from build123d import *

# Parameters (mm, degrees)
SKETCH003_W     = 161.5
SKETCH003_H     = 211.5
SKETCH003_W_2   = 130
SKETCH003_H_2   = 180
PAD002_DEPTH    = 18.5
SKETCH004_W     = 142.953762
SKETCH004_H     = 192.038153
SKETCH004_W_2   = 116
SKETCH004_H_2   = 167
PAD003_DEPTH    = 7.6
SKETCH011_W     = 36.28281
SKETCH011_H     = 83.99005
POCKET002_DEPTH = 6.5


with BuildPart() as part:
    # Sketch003 (on XY_Plane031 of Origin062) → Pad002 (new body)
    with BuildSketch(Plane.XY):
        with Locations((80.75, 105.75)):
            Rectangle(SKETCH003_W, SKETCH003_H)
        with Locations((80.75, 105.75)):
            Rectangle(SKETCH003_W_2, SKETCH003_H_2, mode=Mode.SUBTRACT)
    extrude(amount=PAD002_DEPTH)

    # Sketch004 (on Face10 of Pad002) → Pad003 (join)
    with BuildSketch(Plane.XY.offset(18.5)):
        with Locations((79.935823, 103.608654)):
            Rectangle(SKETCH004_W, SKETCH004_H)
        with Locations((80.75, 105.75)):
            Rectangle(SKETCH004_W_2, SKETCH004_H_2, mode=Mode.SUBTRACT)
    extrude(amount=-PAD003_DEPTH)

    # Sketch011 (on Face4 of Pad003) → Pocket002 (cut)
    with BuildSketch(Plane(origin=(0, 0, 0), x_dir=(1, 0, 0), z_dir=(0, 0, -1))):
        with Locations((161.891405, -94.345025)):
            Rectangle(SKETCH011_W, SKETCH011_H)
    extrude(amount=-POCKET002_DEPTH, mode=Mode.SUBTRACT)


solid = part.part
Check sheet for the modelled part. Datum: model origin and axes. Units: mm. A direction names the side the tool comes from. Give positions to 0.01 mm unless a question says otherwise; leave off trailing zeros. Write each loop counter-clockwise with the first axis right and the second up, starting at its lowest first coordinate (ties: lowest second). Pieces come first, ordered by that corner, then holes. Notation, with made-up numbers: (-37, -29) -> (-19, -29) arc R3 cw to (-19, -25) -> close; hole circle Ø11 at (57.5, 42.25). An arc over 180 degrees is marked (long way). One line per item, written item: value. Start each with the question number.
Item 1: Section check B-B on x = 110. Record the cut outline in (y, z), then the cut area to 3 significant figures.
Item 2: Section check C-C on y = 19. Record the cut outline in (x, z), then the cut area to 3 significant figures.
Item 3: Gauge pin test, flat ends, axial feed: pin 1 (5.5 mm diameter, centred on x = 53, z = 4.5, fed in from -Y); pin 2 (17.5 mm diameter, centred on x = 154, y = 113, fed in from -Z). Record the tip position at first contact, or that the pin passes through.
Item 4: Tool access check on faces 1 (the flat face through (0, 104, 9)), 2 (the flat face through (80, 22.25, 15)), 3 (the flat face through (80, 15.75, 5)), 4 (the flat face through (154, 52.35, 3)), 5 (the flat face through (8, 107, 18.5)). Record the directions out of +Z, -Z, +X, -X, +Y, -Y that give a thin tool (end or side, any length) a straight path to the whole face; none if there is none.
Item 5: Section check A-A on y = 42.5. Record the cut outline in (x, z).
Item 6: Section check D-D on x = 151.5. Record the cut outline in (y, z).
Item 7: Draft check along X on faces 6 (the flat face through (161.5, 104, 11)), 7 (the flat face through (80, 189.25, 15)), 8 (the flat face through (154, 94, 6.5)). Enter one of: +X half, -X half, draft (parallel to the pull), parting line (faces both ways), or undercut.
Item 8: Material ranges on probe 1 along Y at (x, z) = (88, 16); probe 2 along Y at (x, z) = (119.5, 1); probe 3 along X at (y, z) = (60, 17.25), recorded low to high. Write a range as from..to.
Results list:
1. outline: (0, 0) -> (15.75, 0) -> (15.75, 10.9) -> (22.25, 10.9) -> (22.25, 18.5) -> (0, 18.5) -> close; (189.25, 10.9) -> (195.75, 10.9) -> (195.75, 0) -> (211.5, 0) -> (211.5, 18.5) -> (189.25, 18.5) -> close
1. area: 682 mm²
2. outline: (0, 0) -> (15.75, 0) -> (15.75, 10.9) -> (145.75, 10.9) -> (145.75, 0) -> (161.5, 0) -> (161.5, 18.5) -> (0, 18.5) -> close
2. area: 1,570 mm²
3. pin 1: y = 0
3. pin 2: z = 6.5
4. face 1: +Z, -Z, -X, +Y, -Y
4. face 2: +Z, -Z
4. face 3: -Z
4. face 4: -Z, +X
4. face 5: +Z, +X, -X, +Y, -Y
5. outline: (0, 0) -> (15.75, 0) -> (15.75, 10.9) -> (22.75, 10.9) -> (22.75, 18.5) -> (0, 18.5) -> close; (138.75, 10.9) -> (145.75, 10.9) -> (145.75, 0) -> (161.5, 0) -> (161.5, 18.5) -> (138.75, 18.5) -> close
6. outline: (0, 0) -> (52.35, 0) -> (52.35, 6.5) -> (136.34, 6.5) -> (136.34, 0) -> (211.5, 0) -> (211.5, 18.5) -> (0, 18.5) -> close
7. face 6: +X half
7. face 7: undercut
7. face 8: draft
8. probe 1: 0..22.25, 189.25..211.5
8. probe 2: 0..15.75, 195.75..211.5
8. probe 3: 0..22.75, 138.75..161.5
